Design review of the part shown in the three views and the two pictorial views. Dimensions are in mm from the part's minimum x, y and z. A direction names the side the tool comes from. Give positions to 0.01 mm unless a question says otherwise; leave off trailing zeros. Loops run counter-clockwise (first coordinate to the right, second up) from the corner with the lowest first, then second, coordinate; pieces in that order, holes last. Notation, with made-up numbers: (-4, -29.75) -> (1, -29.75) arc R28 cw to (1, 2.25) -> close; hole circle Ø9 at (20, 81). An arc over 180 degrees is marked (long way). Answer as CSV lines item,"result".
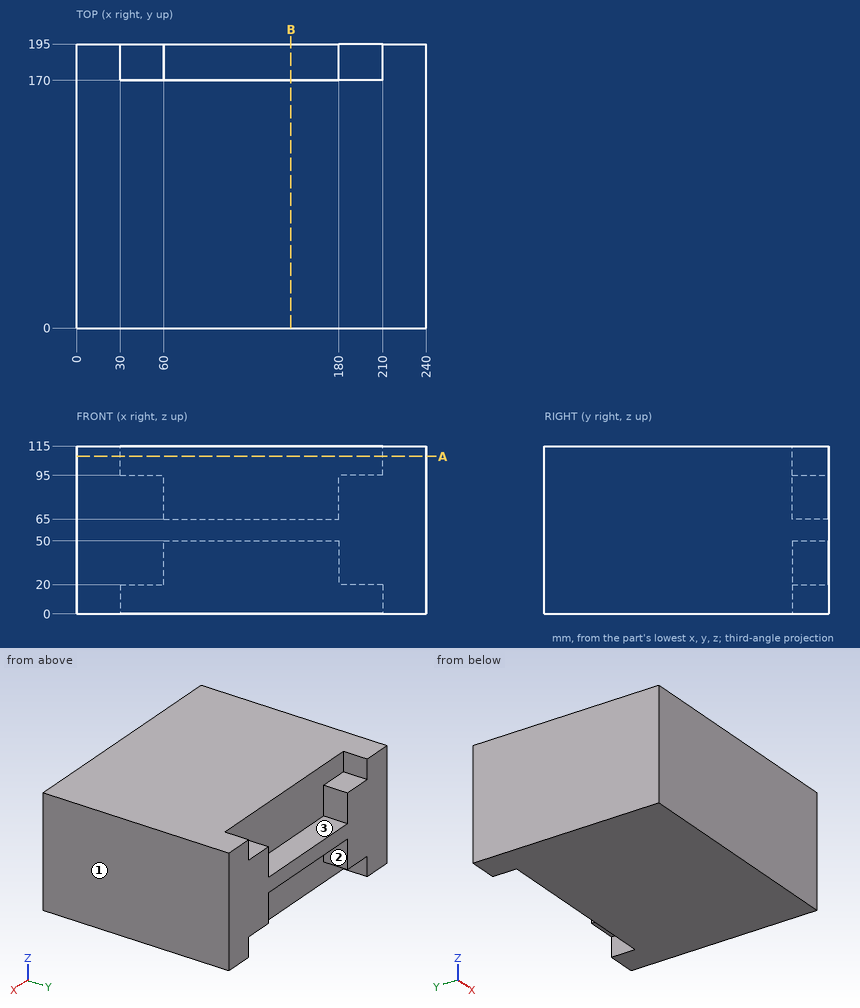
Q1. We need section A-A, the plane z = 108. State the section outline as (x, y) points, and give its area (3 significant figures).
Filled sheet:
outline,"(0, 0) -> (240, 0) -> (240, 195) -> (210, 195) -> (210, 170) -> (30, 170) -> (30, 195) -> (0, 195) -> close"
area,"42,300 mm^2"
Q2. We need section B-B, the plane x = 147. State the section outline as (y, z) points.
Filled sheet:
outline,"(0, 0) -> (170, 0) -> (170, 50) -> (195, 50) -> (195, 65) -> (170, 65) -> (170, 115) -> (0, 115) -> close"
Q3. Clearance check with flat-ended pins moving along their axes: pin 1 Ø12 at (x, z) = (129, 79.5) entering from +Y; pin 2 Ø20 at (x, y) = (137, 181.5) entering from +Z; pin 3 Ø20 at (x, y) = (187.5, 184) entering from +Z. State where each tip first meets the part, or that it passes through.
Filled sheet:
pin 1,"stops at y = 170"
pin 2,"stops at z = 65"
pin 3,"stops at z = 95"
Q4. For the marked faces 1, 2 and 3, list the 3-axis set-ups (+Z, -Z, +X, -X, +Y, -Y) from which the entire face can be reached by the end or side of a thin tool; tool diameter is ignored.
Filled sheet:
face 1,"+Z, -Z, +X, +Y, -Y"
face 2,"-Z, +Y"
face 3,"+Z, +Y"
Q5. To check wall thickness, follow probe 1 along X at (y, z) = (180, 80); probe 2 along Z at (x, y) = (199, 184); probe 3 along Y at (x, z) = (162.5, 86). State the ranges of each line that lie inside material, in increasing order. Write a range as from..to.
Filled sheet:
probe 1,"x = 0..60, 180..240"
probe 2,"z = 20..95"
probe 3,"y = 0..170"
